from build123d import *

# Parameters (mm, degrees)
F0_R          = 8.25
F1_DEPTH      = 25.4
F2_R          = 1.5
F3_DEPTH      = 18.051
F4_SIZE       = 2.54
F5_R          = 1.5
F6_DEPTH      = 2.5
F6_DEPTH_BACK = 25.4


with BuildPart() as f1:
    # F0 (on Front) → F1 (new body)
    with BuildSketch(Plane.XZ):
        with BuildLine():
            Line((-13.4290065467, 14.4366604356), (-21.0230065467, 14.4366604356))
            ThreePointArc((-21.0230065467, 14.4366604356), (-30.9290065467, 24.3426604356), (-40.8350065467, 14.4366604356))
            Line((-40.8350065467, 14.4366604356), (-48.4290065467, 14.4366604356))
            Line((-48.4290065467, 14.4366604356), (-48.4290065467, -3.6133395644))
            Line((-48.4290065467, -3.6133395644), (-13.4290065467, -3.6133395644))
            Line((-13.4290065467, -3.6133395644), (-13.4290065467, 14.4366604356))
        make_face()
        with Locations((-30.9290065467, 14.4366604356)):
            Circle(F0_R, mode=Mode.SUBTRACT)
    extrude(amount=F1_DEPTH)

    # F2 (on face) → F3 (cut, through all)
    with BuildSketch(Plane.XY.offset(14.4366604356)):
        with Locations((-42.9290065467, -21.332904214)):
            Circle(F2_R)
        with Locations((-42.9290065467, -3.332904214)):
            Circle(F2_R)
        with Locations((-18.9290065467, -3.332904214)):
            Circle(F2_R)
        with Locations((-18.9290065467, -20.2919691801)):
            Circle(F2_R)
    extrude(amount=-F3_DEPTH, mode=Mode.SUBTRACT)

    # F4
    f4_edges = [f1.edges().sort_by_distance(p)[0] for p in [
        (-48.429007, -12.7, 14.43666),
        (-13.429007, -12.7, 14.43666),
    ]]
    chamfer(f4_edges, length=F4_SIZE)

    # F5 (on face) → F6 (cut, two sides)
    with BuildSketch(Plane.XY.offset(14.4366604356)) as f6_sk:
        Polygon((-44.6610573543, -6.332904214), (-41.1969557392, -6.332904214), (-39.4649049316, -3.332904214), (-41.1969557392, -0.332904214), (-44.6610573543, -0.332904214), (-46.3931081619, -3.332904214), align=None)
        with Locations((-42.9290065467, -3.332904214)):
            Circle(F5_R, mode=Mode.SUBTRACT)
        Polygon((-44.6610573543, -24.332904214), (-41.1969557392, -24.332904214), (-39.4649049316, -21.332904214), (-41.1969557392, -18.332904214), (-44.6610573543, -18.332904214), (-46.3931081619, -21.332904214), align=None)
        with Locations((-42.9290065467, -21.332904214)):
            Circle(F5_R, mode=Mode.SUBTRACT)
        Polygon((-20.6610573543, -6.332904214), (-17.1969557392, -6.332904214), (-15.4649049316, -3.332904214), (-17.1969557392, -0.332904214), (-20.6610573543, -0.332904214), (-22.3931081619, -3.332904214), align=None)
        with Locations((-18.9290065467, -3.332904214)):
            Circle(F5_R, mode=Mode.SUBTRACT)
        Polygon((-20.6610573543, -23.2919691801), (-17.1969557392, -23.2919691801), (-15.4649049316, -20.2919691801), (-17.1969557392, -17.2919691801), (-20.6610573543, -17.2919691801), (-22.3931081619, -20.2919691801), align=None)
        with Locations((-18.9290065467, -20.2919691801)):
            Circle(F5_R, mode=Mode.SUBTRACT)
    extrude(amount=-F6_DEPTH, mode=Mode.SUBTRACT)
    extrude(f6_sk.sketch, amount=F6_DEPTH_BACK, mode=Mode.SUBTRACT)


solid = f1.part
Check sheet for the modelled part. Datum: model origin and axes. Units: mm. A direction names the side the tool comes from. Round coordinates to 2 decimals unless told otherwise and drop trailing zeros. Order: outer loops, then holes, each group sorted by start corner. A loop starts at its lowest first (then second) coordinate and runs counter-clockwise, first axis right, second up.
(1) Draft check along X on faces 4 (the flat face through (-48.429, -13, 4)), 5 (the flat face through (-18, -24, 14.437)), 6 (the flat face through (-45.515, -1.812, 13.204)). Enter one of: pulls with the +X half, pulls with the -X half, needs draft (parallel to the pull), parting line crosses it, or undercut.
(2) Cross-section at D-D, the plane y = -15.25. Enter the section's corners in (x, z) (3 decimals), and give its area (3 significant figures).
(3) Access from +Z, -Z, +X, -X, +Y, -Y to the whole of each face (thin tool, end or side, straight path). Record for faces 1 (the flat face through (-16.32, -1.85, 13.2)), 2 (the flat face through (-18, -12, 14.437)), 3 (the flat face through (-31, -25.4, 4)).
(4) Go/stop test with flat-tipped pins: P1, Ø10, axis at x = -20.5, y = -17, coming from the +Z side; P2, Ø5, axis at x = -42.93, y = -3.33, coming from the -Z side; P3, Ø2.5, axis at x = -19, y = -1, coming from the +Z side; P4, Ø8, axis at y = -17, z = 18.5, coming from the +X side. Record where each tip stops, or that it passes through.
(5) Cross-section at C-C, the plane x = -24.5. Enter the section's corners in (y, z).
(6) Scan lines: probe 1 along X at (y, z) = (-21.5, 10); probe 2 along X at (y, z) = (-22.75, 12.5); probe 3 along Z at (x, y) = (-17.5, -5.25). Record each from-to range of solid material in increasing order.
(7) Cross-section at B-B, the plane z = 5. Enter the section's corners in (x, y), and give its area (3 significant figures).
(8) Cross-section at A-A, the plane z = 8.5. Enter the section's corners in (x, y).
Check sheet entries:
1. face 4: pulls with the -X half
1. face 5: needs draft
1. face 6: undercut
2. outline: (-48.429, -3.613) - (-13.429, -3.613) - (-13.429, 11.897) - (-15.969, 14.437) - (-21.023, 14.437) arc R9.906 ccw to (-40.835, 14.437) - (-45.889, 14.437) - (-48.429, 11.897) - close; hole circle Ø16.5 at (-30.929, 14.437)
2. area: 566 mm2
3. face 1: +Z
3. face 2: +Z, +X, +Y, -Y
3. face 3: +Z, -Z, +X, -X, -Y
4. P1: stops at z = 22.72
4. P2: stops at z = -3.61
4. P3: stops at z = 14.44
4. P4: stops at x = -21.02
5. outline: (-25.4, -3.61) - (0, -3.61) - (0, 9.27) - (-25.4, 9.27) - close; (-25.4, 19.61) - (0, 19.61) - (0, 21.97) - (-25.4, 21.97) - close
6. probe 1: x = -48.43 to -44.42, -41.44 to -37.88, -23.97 to -19.82, -18.04 to -13.43
6. probe 2: x = -47.83 to -45.57, -40.28 to -38.95, -22.91 to -20.97, -16.88 to -14.03
6. probe 3: z = -3.61 to 11.94
7. outline: (-48.43, -25.4) - (-13.43, -25.4) - (-13.43, 0) - (-48.43, 0) - close; hole circle Ø3 at (-42.93, -21.33); hole circle Ø3 at (-42.93, -3.33); hole circle Ø3 at (-18.93, -20.29); hole circle Ø3 at (-18.93, -3.33)
7. area: 861 mm2
8. outline: (-48.43, -25.4) - (-36.66, -25.4) - (-36.66, 0) - (-48.43, 0) - close; (-25.2, -25.4) - (-13.43, -25.4) - (-13.43, 0) - (-25.2, 0) - close; hole circle Ø3 at (-42.93, -21.33); hole circle Ø3 at (-42.93, -3.33); hole circle Ø3 at (-18.93, -20.29); hole circle Ø3 at (-18.93, -3.33)
